from build123d import *

# Parameters (mm, degrees)
BOSS_EXTRUDE1_DEPTH = 15
SKETCH2_R           = 3
CUT_EXTRUDE1_DEPTH  = 59.949130613
SKETCH3_W           = 70
SKETCH3_H           = 10
BOSS_EXTRUDE2_DEPTH = 10
SKETCH4_R           = 6
CUT_EXTRUDE2_DEPTH  = 7


with BuildPart() as part:
    # Sketch1 → Boss-Extrude1 (new body)
    with BuildSketch(Plane(origin=(0, 0, 0), x_dir=(0, 0, -1), z_dir=(1, 0, 0))):
        with BuildLine():
            Line((16, 45), (35, 45))
            Line((35, 45), (35, 0))
            Line((35, 0), (-35, 0))
            Line((-35, 0), (-35, 45))
            Line((-35, 45), (-16, 45))
            ThreePointArc((-16, 45), (0, 29), (16, 45))
        make_face()
    extrude(amount=BOSS_EXTRUDE1_DEPTH)

    # Sketch2 → Cut-Extrude1 (cut, through all)
    with BuildSketch(Plane(origin=(0, 0, 0), x_dir=(1, 0, 0), z_dir=(0, 1, 0))):
        with Locations(Location((10, -27, 0), (0, 0, 90))):
            Circle(SKETCH2_R)
        with Locations(Location((10, 27, 0), (0, 0, 90))):
            Circle(SKETCH2_R)
    extrude(amount=CUT_EXTRUDE1_DEPTH, mode=Mode.SUBTRACT)

    # Sketch3 → Boss-Extrude2 (add)
    with BuildSketch(Plane(origin=(15, 0, 0), x_dir=(0, 0, -1), z_dir=(1, 0, 0))):
        with Locations((0, 5)):
            Rectangle(SKETCH3_W, SKETCH3_H)
    extrude(amount=BOSS_EXTRUDE2_DEPTH)

    # Sketch4 → Cut-Extrude2 (cut)
    with BuildSketch(Plane.XZ):
        with Locations(Location((10, 27, 0), (0, 0, 270))):
            Circle(SKETCH4_R)
        with Locations(Location((10, -27, 0), (0, 0, 270))):
            Circle(SKETCH4_R)
    extrude(amount=-CUT_EXTRUDE2_DEPTH, mode=Mode.SUBTRACT)


solid = part.part
CAD build for the part. Positions are in the model's coordinates, mm. A direction names the side the tool comes from. Coordinates: 2 decimals unless noted, no trailing zeros. Loops run counter-clockwise (first coordinate to the right, second up) from the corner with the lowest first, then second, coordinate; pieces in that order, holes last. Notation, with made-up numbers: (9, 79.25) - (25, 79.25) arc R18 cw to (25, 111.25) - close; hole circle Ø11 at (28, 2). An arc over 180 degrees is marked (long way). Use one line per item in the form item = value. Start each with the question number.
1) Band-saw the part on D-D (x = 6.25). Give the cut face in (y, z), and give its area (3 significant figures).
2) Flat gauge pins, fed straight in: pin 1 (9.5 mm diameter, centred on x = 10, z = -27, fed in from -Y); pin 2 (17.5 mm diameter, centred on y = 24, z = -14.5, fed in from +X); pin 3 (3 mm diameter, centred on x = 19.5, z = -14, fed in from +Y). Where does each tip first touch, or does it go through?
3) Drill centre lines: L1, parallel to X at y = 4, z = 27; L2, parallel to X at y = 16, z = 27; L3, parallel to Z at x = 7.25, y = 39.5. Where is each one in solid material? Low to high. Write a range as from..to.
4) Band-saw the part on A-A (z = 27). Give the cut face in (x, y), and give its area (3 significant figures).
5) Band-saw the part on B-B (y = 37). Give the cut face in (x, z).
6) Band-saw the part on C-C (y = 13). Give the cut face in (x, z), and give its area (3 significant figures).
7) Tool access for faces 4 (the face through (15, 24, 0)), 5 (the face through (6.35, 3.45, -22.24)), 6 (the face through (7, 29, 0)): list every direction of +Z, -Z, +X, -X, +Y, -Y with a clear straight run to the whole face (end or side of a thin tool).
8) Two-plate mould, pull along Z, no slides. Class faces 1 (the face through (10, 17, -35)), 2 (the face through (10, 26, -24)), 3 (the face through (0, 23, 0)): +Z half, -Z half, draft (parallel to the pull), parting line (faces both ways), or undercut.
Check values:
q1.outline = (0, -35) - (45, -35) - (45, -16) arc R16 cw to (45, 16) - (45, 35) - (0, 35) - (0, 31.68) - (7, 31.68) - (7, 22.32) - (0, 22.32) - (0, -22.32) - (7, -22.32) - (7, -31.68) - (0, -31.68) - close
q1.area = 2,620 mm2
q2.pin_1 = 7
q2.pin_2 = 15
q2.pin_3 = 10
q3.L1 = 0..4, 16..25
q3.L2 = 0..7, 13..15
q3.L3 = -35..-28.2, -25.8..-15.02, 15.02..25.8, 28.2..35
q4.outline = (0, 0) - (4, 0) - (4, 7) - (7, 7) - (7, 45) - (0, 45) - close; (13, 7) - (16, 7) - (16, 0) - (25, 0) - (25, 10) - (15, 10) - (15, 45) - (13, 45) - close
q4.area = 463 mm2
q5.outline = (0, -35) - (15, -35) - (15, -13.86) - (0, -13.86) - close; (0, 13.86) - (15, 13.86) - (15, 35) - (0, 35) - close; hole circle Ø6 at (10, -27); hole circle Ø6 at (10, 27)
q6.outline = (0, -35) - (15, -35) - (15, 35) - (0, 35) - close; hole circle Ø6 at (10, -27); hole circle Ø6 at (10, 27)
q6.area = 993 mm2
q7.face_4 = +Z, -Z, +X, +Y
q7.face_5 = -Y
q7.face_6 = +X, -X, +Y
q8.face_1 = -Z half
q8.face_2 = undercut
q8.face_3 = draft
